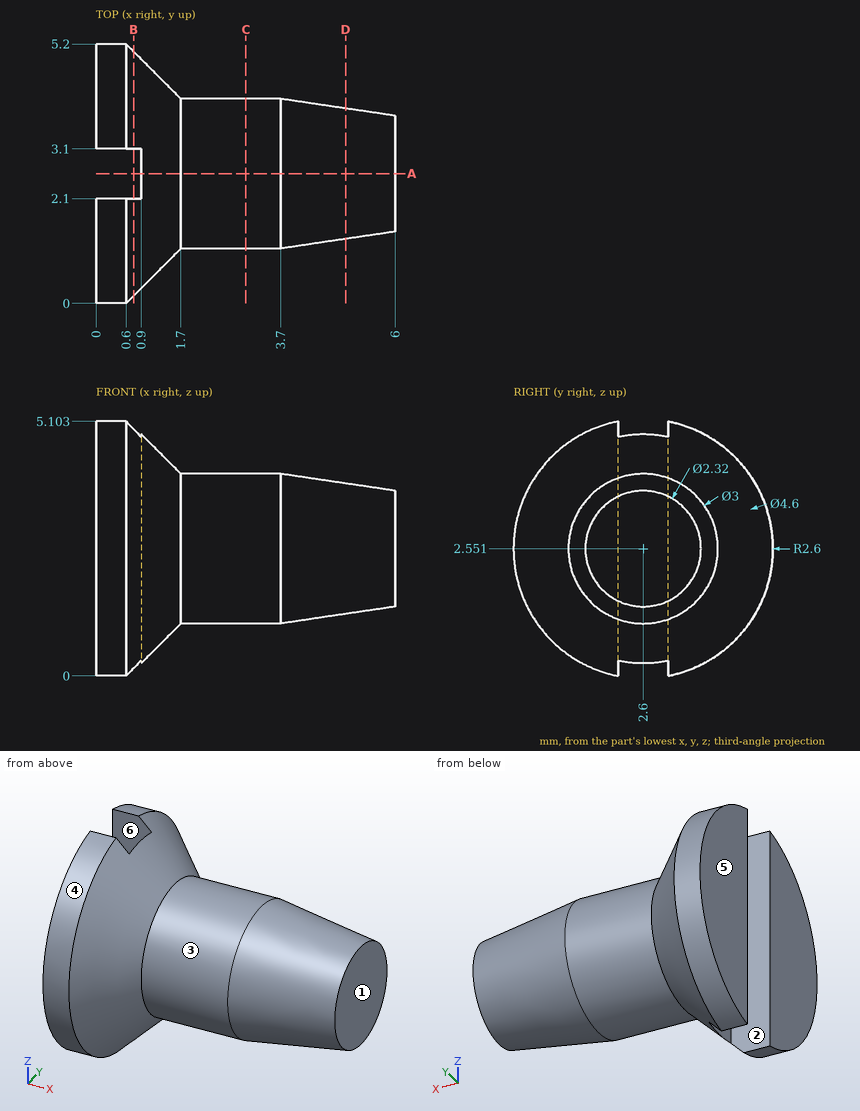
The drawing under review shows one solid part. Ordinate dimensions are in mm from its lowest x, y, z. A direction names the side the tool comes from. Round coordinates to 2 decimals unless told otherwise and drop trailing zeros. Write each loop counter-clockwise with the first axis right and the second up, starting at its lowest first coordinate (ties: lowest second). Pieces come first, ordered by that corner, then holes.
(1) We need section C-C on x = 3. Give the boundary of the cut face in (y, z).
(2) Insertion check: pin 1 (0.5 mm diameter, centred on y = 2.5, z = 2.5, fed in from -X); pin 2 (1 mm diameter, centred on y = 2, z = 3.5, fed in from -X); pin 3 (1 mm diameter, centred on y = 4.5, z = 1, fed in from +X); pin 4 (0.5 mm diameter, centred on x = 0.5, z = 3.5, fed in from -Y) (1 decimal). Each pin has a flat end and moves straight along its axis. Give the tip position at first contact, or say it passes through.
(3) Machinability: for the marked faces 1, 2 and 3, which of the approach directions +Z, -Z, +X, -X, +Y, -Y give a long, thin tool a straight path to every point of the face, cutting with its end or side? Answer none if there is none.
(4) We need section B-B on x = 0.75. Give the boundary of the cut face in (y, z), and give its area (3 significant figures).
(5) Wall thickness on L1, parallel to Z at x = 3, y = 3.55; L2, parallel to Y at x = 3.5, z = 1.6; L3, parallel to Z at x = 0.5, y = 4.05 (1 decimal): over which ranges is each line inside the solid? List them lowest first.
(6) We need section D-D on x = 5. Give the boundary of the cut face in (y, z) (1 decimal).
(7) We need section A-A on y = 2.6. Give the boundary of the cut face in (x, z).
(8) Mouldability with a two-part tool opening along Y and no side actions: class the marked faces 4, 5 and 6 as +Y half, -Y half, draft (parallel to the pull), parting line (faces both ways), or undercut.
Findings below:
1. outline: circle Ø3 at (2.6, 2.55)
2. pin 1: stops at x = 0.9
2. pin 2: stops at x = 0
2. pin 3: stops at x = 1.25
2. pin 4: stops at y = 0.1
3. face 1: +Z, -Z, +X, +Y, -Y
3. face 2: +Z, -Z, -X
3. face 3: +X
4. outline: (2.1, 0.15) - (2.1, 4.95) arc R2.45 ccw to start; (3.1, 0.15) arc R2.45 ccw to (3.1, 4.95) - close
4. area: 14.0 mm2
5. L1: z = 1.39 to 3.71
5. L2: y = 1.44 to 3.76
5. L3: z = 0.4 to 4.7
6. outline: circle Ø2.6 at (2.6, 2.6)
7. outline: (0.9, 0.25) - (1.7, 1.05) - (3.7, 1.05) - (6, 1.39) - (6, 3.71) - (3.7, 4.05) - (1.7, 4.05) - (0.9, 4.85) - close
8. face 4: -Y half
8. face 5: draft
8. face 6: undercut
